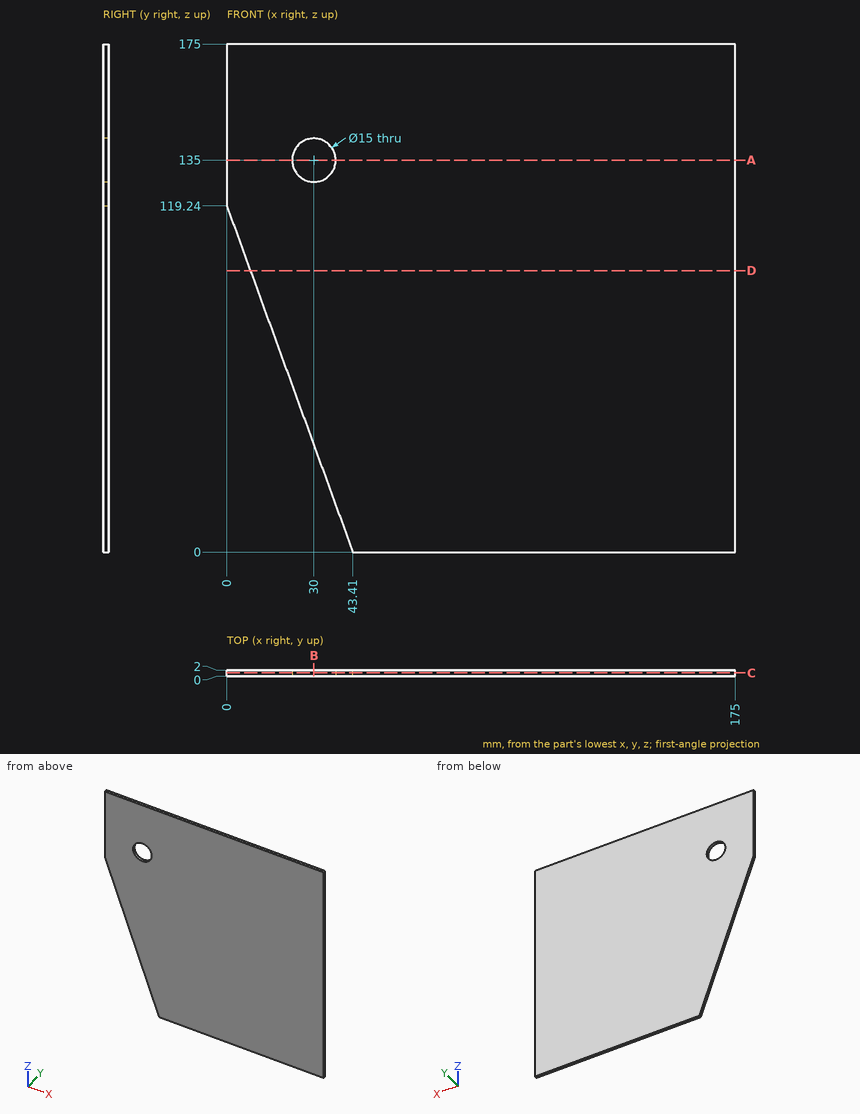
Verification items for this drawing (mm, ordinates from the low corner). Coordinates: 2 decimals unless noted, no trailing zeros. Write each loop counter-clockwise with the first axis right and the second up, starting at its lowest first coordinate (ties: lowest second). Pieces come first, ordered by that corner, then holes. Notation, with made-up numbers: M 81,31 L 130,31 A25 cw 130,65 Z; hole C 35.25,-14 d11. An arc over 180 degrees is marked long. One line per item, written item: value. Start each with the question number.
(1) Scan lines: line 1 along X through (y, z) = (1.1, 135); line 2 along X through (y, z) = (0.5, 82.5); line 3 along X through (y, z) = (0.5, 54.5). Record each from-to range of solid material in increasing order. Write a range as [from, to].
(2) Sectioned sample at B-B, the plane x = 30. Enter the section's corners in (y, z), and give its area (3 significant figures).
(3) Sectioned sample at C-C, the plane y = 1.05. Enter the section's corners in (x, z).
(4) Sectioned sample at D-D, the plane z = 97. Enter the section's corners in (x, y).
(5) Sectioned sample at A-A, the plane z = 135. Enter the section's corners in (x, y).
Filled sheet:
1. line 1: [0, 22.5], [37.5, 175]
1. line 2: [13.38, 175]
1. line 3: [23.57, 175]
2. outline: M 0,36.84 L 2,36.84 L 2,127.5 L 0,127.5 Z; M 0,142.5 L 2,142.5 L 2,175 L 0,175 Z
2. area: 246 mm²
3. outline: M 0,119.24 L 43.41,0 L 175,0 L 175,175 L 0,175 Z; hole C 30,135 d15
4. outline: M 8.1,0 L 175,0 L 175,2 L 8.1,2 Z
5. outline: M 0,0 L 22.5,0 L 22.5,2 L 0,2 Z; M 37.5,0 L 175,0 L 175,2 L 37.5,2 Z
